from build123d import *

# Parameters (mm, degrees)
F0_W     = 76.2
F0_H     = 38.1
F1_DEPTH = 25.4
F2_W     = 12.7
F2_H     = 6.35
F3_DEPTH = 36.83
F4_W     = 12.7
F4_H     = 6.35
F5_DEPTH = 101.854


with BuildPart() as f1:
    # F0 (on Front) → F1 (new body)
    with BuildSketch(Plane.XZ):
        Rectangle(F0_W, F0_H)
    extrude(amount=F1_DEPTH)

    # F2 (on Front) → F3 (cut)
    with BuildSketch(Plane.XZ):
        with Locations((-28.330677, 12.612414)):
            Rectangle(F2_W, F2_H)
    extrude(amount=-F3_DEPTH, mode=Mode.SUBTRACT)

    # F4 (on Front) → F5 (cut)
    with BuildSketch(Plane.XZ):
        with Locations((-24.622671, 14.386035)):
            Rectangle(F4_W, F4_H)
    extrude(amount=F5_DEPTH, mode=Mode.SUBTRACT)


solid = f1.part
Can you work these out from the model? Positions are in its coordinate system, mm. A direction names the side the tool comes from. Round coordinates to 2 decimals unless told otherwise and drop trailing zeros. Loops run counter-clockwise (first coordinate to the right, second up) from the corner with the lowest first, then second, coordinate; pieces in that order, holes last. Notation, with made-up numbers: (76.5, 55.5) - (85.5, 55.5) arc R29 ccw to (85.5, 90.5) - close; hole circle Ø1 at (78, 82.25). An arc over 180 degrees is marked (long way). Use CSV: the item, a comma, the result in double quotes. Start each with the question number.
1) We'd pull the mould along X, two halves only. Please class faces 3 (the flat face through (-1, -13, -19.05)), 4 (the flat face through (38.1, -13, 0)), 5 (the flat face through (-38.1, -13, 0)), 6 (the flat face through (-25, -13, 17.561)): released by +X, released by -X, zero draft, split by the parting line, or undercut.
2) Please list where these lines run through material, in increasing order: probe 1 along X at (y, z) = (-7.5, 11.5); probe 2 along Z at (x, y) = (-24, -16.25). Write a range as [from, to].
3) If we section it at B-B on z = 16: Write out the boundary of the cut face in (x, y), plus the area to 3 significant figures.
4) For pin 1 Ø5 at (x, z) = (19, 9.5) entering from +Y, with a flat end and sliding along its axis, tell me the tip position at first contact or that it passes through.
5) If we section it at A-A on x = -26: Write out the boundary of the cut face in (y, z).
6) If we section it at C-C on y = -3: Write out the boundary of the cut face in (x, z), plus the area to 3 significant figures.
7) For faces 1 (the flat face through (-1, -13, 19.05)), 2 (the flat face through (-18.273, -13, 14)), which set-ups out of +Z, -Z, +X, -X, +Y, -Y let a thin tool reach every point of the face, with its end or its side?
Geometry results:
1,face 3,"zero draft"
1,face 4,"released by +X"
1,face 5,"released by -X"
1,face 6,"undercut"
2,probe 1,"x = [-38.1, -30.97], [-18.27, 38.1]"
2,probe 2,"z = [-19.05, 11.21], [17.56, 19.05]"
3,outline,"(-38.1, -25.4) - (-30.97, -25.4) - (-30.97, 0) - (-38.1, 0) - close; (-18.27, -25.4) - (38.1, -25.4) - (38.1, 0) - (-18.27, 0) - close"
3,area,"1,610 mm2"
4,pin 1,"stops at y = 0"
5,outline,"(-25.4, -19.05) - (0, -19.05) - (0, 11.21) - (-25.4, 11.21) - close; (-25.4, 17.56) - (0, 17.56) - (0, 19.05) - (-25.4, 19.05) - close"
6,outline,"(-38.1, -19.05) - (38.1, -19.05) - (38.1, 19.05) - (-38.1, 19.05) - close; hole (-30.97, 11.21) - (-18.27, 11.21) - (-18.27, 17.56) - (-30.97, 17.56) - close"
6,area,"2,820 mm2"
7,face 1,"+Z, +X, -X, +Y, -Y"
7,face 2,"+Y, -Y"
